CAD build for the part. Positions are in the model's coordinates, mm. Face numbers are marked on the shaded views. A direction names the side the tool comes from. Round coordinates to 2 decimals unless told otherwise and drop trailing zeros. Loops run counter-clockwise (first coordinate to the right, second up) from the corner with the lowest first, then second, coordinate; pieces in that order, holes last.
Autodesk Inventor part; units mm, degrees
ref_plane "YZ Plane" through (0, 0, 0) normal (1, 0, 0) x (0, 1, 0)
ref_plane "XZ Plane" through (0, 0, 0) normal (0, 1, 0) x (-1, 0, 0)
ref_plane "XY Plane" through (0, 0, 0) normal (0, 0, 1) x (1, 0, 0)
sketch "Sketch1" plane through (0, 0, 0) normal (0, 0, 1) x (1, 0, 0)
  line L0 (0, 0) -> (47, 0)
  line L1 (47, 10.25) -> (0, 10.25)
  line L2 (0, 10.25) -> (0, 17.75)
  line L3 (47, 10.25) -> (47, 23.25)
  line L4 (47, 23.25) -> (17, 23.25)
  line L5 (17, 23.25) -> (17, 86.75)
  line L6 (17, 86.75) -> (25.6776, 97.0916)
  line L7 (25.6776, 97.0916) -> (27.4678, 104.8887)
  line L8 (27.4678, 104.8887) -> (27.4678, 117.8887)
  line L9 (27.4678, 117.8887) -> (26.1178, 117.8887)
  line L10 (26.1178, 117.8887) -> (22.9803, 105.273)
  line L11 (22.9803, 105.273) -> (16.9803, 105.273)
  line L12 (16.9803, 105.273) -> (13.8419, 117.8885)
  line L13 (13.8419, 117.8885) -> (12.4919, 117.8885)
  line L14 (12.4919, 117.8885) -> (9.3536, 105.273)
  line L15 (9.3536, 105.273) -> (3.3536, 105.273)
  line L16 (0, 117.8885) -> (1.35, 117.8885)
  line L17 (1.35, 117.8885) -> (3.3536, 105.273)
  line L18 (0, 117.8885) -> (0, 103.8885)
  line L19 (0, 103.8885) -> (2.2376, 94.1421)
  line L20 (2.2376, 94.1421) -> (10.2376, 94.1421)
  line L21 (0, 17.75) -> (10.2376, 24.25)
  line L22 (10.2376, 94.1421) -> (10.2376, 24.25)
  dimension "d0" = 47
  dimension "d1" = 10.25
  dimension "d3" = 7.5
  dimension "d4" = 13
  dimension "d27" = 30
  dimension "d28" = 63.5
  dimension "d34" = 13.5
  dimension "d35" = 140
  dimension "d36" = 8
  dimension "d37" = 13
  dimension "d38" = 1.35
  dimension "d39" = 13
  dimension "d40" = 4.4875
  dimension "d41" = 6
  dimension "d42" = 13
  dimension "d43" = 103.97
  dimension "d44" = 1.35
  dimension "d47" = 13
  dimension "d48" = 6
  dimension "d49" = 103.97
  dimension "d51" = 1.35
  dimension "d52" = 14
  dimension "d53" = 10
  dimension "d54" = 167.07
  dimension "d55" = 8
revolve "Revolution1" add sketch "Sketch1" angle 360 about axis through (0, 0, 0) along (1, 0, 0)
sketch "Sketch2" plane through (0, 0, 0) normal (-1, 0, 0) x (0, 0, 1)
  circle A0 centre (0, 0) radius 17.75
  line L0 (-3.5, 13.75) -> (3.5, 13.75)
  line L1 (3.5, 13.75) -> (3.5, 9.75)
  line L2 (3.5, 9.75) -> (-3.5, 9.75)
  line L3 (-3.5, 9.75) -> (-3.5, 13.75)
  dimension "d61" = 7
  dimension "d62" = 4
extrude "Extrusion1" cut sketch "Sketch2" against normal blind 50 contours L0 L1 L2 L3
properties part number "polia final"
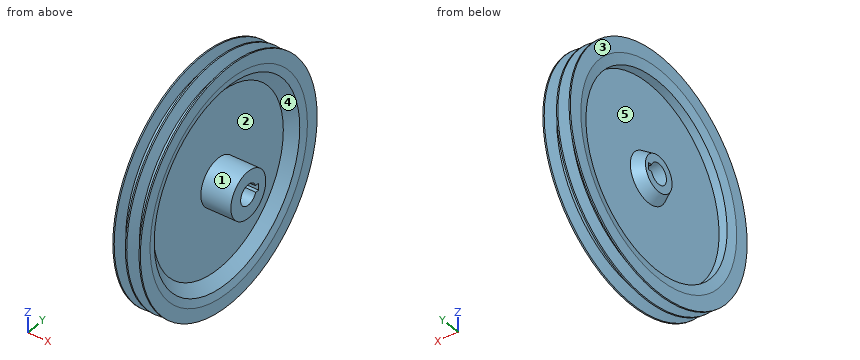
Item 1: Flat gauge pins, fed straight in: P1, Ø2, axis at y = -84, z = -52, coming from the +X side; P2, Ø2, axis at x = 26, y = 12, coming from the -Z side; P3, Ø12, axis at x = 24, z = -40.5, coming from the -Y side. Where does each tip first touch, or does it go through?
Answers follow:
P1: stops at x = 26.3
P2: stops at z = -117.37
P3: stops at y = -112.61
Item 2: Cut at A-A, the plane x = 43. Give the cut face in (y, z), plus the area to 3 significant figures.
Answers follow:
outline: circle Ø46.5 at (0, 0); hole (9.75, -3.5) - (13.75, -3.5) - (13.75, 3.5) - (9.75, 3.5) - (9.75, 3.16) arc R10.25 ccw (long way) to (9.75, -3.16) - close
area: 1,340 mm2
Item 3: Probe line 1 (Z direction, x = 5, y = 0); line 2 (Y direction, x = 18.5, z = 12); line 3 (Z direction, x = 8, y = 0). List the from-to ranges inside material, lowest first.
Answers follow:
line 1: z = -105.27 to -94.14, -20.92 to -10.25, 10.25 to 20.92, 94.14 to 105.27
line 2: y = -104.59 to -87.72, -19.91 to 19.91, 87.72 to 104.59
line 3: z = -105.27 to -94.14, -22.83 to -10.25, 10.25 to 22.83, 94.14 to 105.27
Item 4: 3-axis set-ups, long thin cutter, end or side, ignore diameter. For the marked faces 4 and 5: which of +Z, -Z, +X, -X, +Y, -Y reach the whole face in a straight line?
Answers follow:
face 4: +X
face 5: -X
Item 5: Two-plate mould, pull along Y, no slides. Class the marked faces 1, 2 and 3: released by +Y, released by -Y, zero draft, split by the parting line, or undercut.
Answers follow:
face 1: undercut
face 2: undercut
face 3: zero draft
